```python
from build123d import *

# Parameters (mm, degrees)
SM_BASE_FLANGE_1_DEPTH = 270
SKETCH_2_R             = 2
CUT_EXTRUDE_1_DEPTH    = 10


# Sheet-metal steps are written as plain solids
with BuildPart() as part:
    # Sketch 1 → Базовая кромка1 (new body)
    with BuildSketch(Plane(origin=(0, 0, 0), x_dir=(1, 0, 0), z_dir=(0, 1, 0))):
        with BuildLine():
            Line((-190.103499123, -50.5), (-178.600555398, -50.5))
            ThreePointArc((-178.600555398, -50.5), (-178.141335279, -50.408655439), (-177.75202726, -50.148528137))
            Line((-177.75202726, -50.148528137), (-171.247864204, -43.644365081))
            ThreePointArc((-171.247864204, -43.644365081), (-170.534132837, -43.167465028), (-169.692229286, -43))
            Line((-169.692229286, -43), (-14.007193009, -43))
            ThreePointArc((-14.007193009, -43), (-13.165289458, -43.167465028), (-12.451558091, -43.644365081))
            Line((-12.451558091, -43.644365081), (-1.947395035, -54.148528137))
            ThreePointArc((-1.947395035, -54.148528137), (-1.558087016, -54.408655439), (-1.098866897, -54.5))
            Line((-1.098866897, -54.5), (10.404076828, -54.5))
            Line((10.404076828, -54.5), (10.404076828, -55.5))
            Line((10.404076828, -55.5), (-1.098866897, -55.5))
            ThreePointArc((-1.098866897, -55.5), (-1.940770449, -55.332534972), (-2.654501816, -54.855634919))
            Line((-2.654501816, -54.855634919), (-13.158664872, -44.351471863))
            ThreePointArc((-13.158664872, -44.351471863), (-13.547972891, -44.091344561), (-14.007193009, -44))
            Line((-14.007193009, -44), (-169.692229286, -44))
            ThreePointArc((-169.692229286, -44), (-170.151449405, -44.091344561), (-170.540757423, -44.351471863))
            Line((-170.540757423, -44.351471863), (-177.044920479, -50.855634919))
            ThreePointArc((-177.044920479, -50.855634919), (-177.758651847, -51.332534972), (-178.600555398, -51.5))
            Line((-178.600555398, -51.5), (-190.103499123, -51.5))
            Line((-190.103499123, -51.5), (-190.103499123, -50.5))
        make_face()
    extrude(amount=SM_BASE_FLANGE_1_DEPTH)

    # Эскиз2 → Вырез-Вытянуть1 (cut)
    with BuildSketch(Plane.XY.offset(44)):
        with Locations((-141.849711148, 5)):
            Circle(SKETCH_2_R)
        with Locations((-41.849711148, 5)):
            Circle(SKETCH_2_R)
    extrude(amount=-CUT_EXTRUDE_1_DEPTH, mode=Mode.SUBTRACT)


solid = part.part
```
Here's how the part is built. I have some questions about the finished solid (model axes, mm). A direction names the side the tool comes from. Coordinates: 2 decimals unless noted, no trailing zeros. Loops run counter-clockwise (first coordinate to the right, second up) from the corner with the lowest first, then second, coordinate; pieces in that order, holes last. Notation, with made-up numbers: M -28.75,78.5 L 28.25,78.5 A23 cw 28.25,110.5 Z; hole C 64,-1 d6. An arc over 180 degrees is marked long. One line per item, written item: value.
1. Please list where these lines run through material, in increasing order: probe 1 along Z at (x, y) = (-44.5, 124.5); probe 2 along X at (y, z) = (250, 46); probe 3 along X at (y, z) = (250.5, 50.75).
Geometry says:
probe 1: z = 43 to 44
probe 2: x = -173.6 to -172.19, -11.51 to -10.1
probe 3: x = -190.1 to -176.94, -6.76 to -5.35
2. Thinking about a two-plate mould opening in X: for faces 1 (the flat face through (-89.4, 270, 43.7)), 2 (the flat face through (-7.273, 133.11, 48.823)), 3 (the flat face through (-7.83, 133.11, 49.68)), which applies, +X half, -X half, draft (parallel to the pull), parting line (faces both ways), or undercut?
Geometry says:
face 1: draft
face 2: +X half
face 3: undercut
3. On a 3-axis mill with a long thin cutter (end or side, diameter ignored), from which of +Z, -Z, +X, -X, +Y, -Y can I reach the whole of each face in a straight line? I mean faces 4 (the flat face through (-184, 133, 51.5)), 5 (the flat face through (-184, 133, 50.5)), 6 (the flat face through (-173.75, 133.11, 47.56)), 7 (the flat face through (5, 133, 54.5)), 8 (the flat face through (-93, 133, 43)). Say none if no direction works.
Geometry says:
face 4: +Z, -X, +Y, -Y
face 5: -Z, -X, +Y, -Y
face 6: +Z, +Y, -Y
face 7: -Z, +X, +Y, -Y
face 8: -Z, +X, -X, +Y, -Y
4. Imagine slicing it at C-C (x = -51.5). List the corners of the cut face in (y, z) for me.
Geometry says:
outline: M 0,43 L 270,43 L 270,44 L 0,44 Z
5. Imagine slicing it at A-A (z = 48). List the corners of the cut face in (x, y) for me.
Geometry says:
outline: M -175.6,0 L -174.19,0 L -174.19,270 L -175.6,270 Z; M -9.51,0 L -8.1,0 L -8.1,270 L -9.51,270 Z
6. Will these pins go through, and if not, where does the flat tip stop? pin 1 Ø3.5 at (x, y) = (-187, 137) entering from -Z; pin 2 Ø12.5 at (x, y) = (-182.5, 141.5) entering from +Z; pin 3 Ø2 at (y, z) = (166, 46.5) entering from -X.
Geometry says:
pin 1: stops at z = 50.5
pin 2: stops at z = 51.5
pin 3: stops at x = -175.1
7. Imagine slicing it at B-B (y = 218.5). List the corners of the cut face in (x, z) for me, and give its area (3 significant figures).
Geometry says:
outline: M -190.1,50.5 L -178.6,50.5 A1.2 cw -177.75,50.15 L -171.25,43.64 A2.2 ccw -169.69,43 L -14.01,43 A2.2 ccw -12.45,43.64 L -1.95,54.15 A1.2 cw -1.1,54.5 L 10.4,54.5 L 10.4,55.5 L -1.1,55.5 A2.2 ccw -2.65,54.86 L -13.16,44.35 A1.2 cw -14.01,44 L -169.69,44 A1.2 cw -170.54,44.35 L -177.04,50.86 A2.2 ccw -178.6,51.5 L -190.1,51.5 Z
area: 208 mm2
